Part model, mm, in its own coordinate system. Face numbers are marked on the shaded views. A direction names the side the tool comes from. Give positions to 0.01 mm unless a question says otherwise; leave off trailing zeros. Order: outer loops, then holes, each group sorted by start corner. A loop starts at its lowest first (then second) coordinate and runs counter-clockwise, first axis right, second up.
1. Probe line 1 (Y direction, x = -3.3, z = 7); line 2 (X direction, y = 2.5, z = -8.25); line 3 (X direction, y = 2, z = 7.5). List the from-to ranges inside material, lowest first.
2. Which spindle directions (+Z, -Z, +X, -X, +Y, -Y) get a long thin tool onto all of the face, cutting with end or side? Do the marked faces 1, 2 and 3. Say none if no direction does.
3. Slice it at A-A on z = 5. List the corners of the cut face in (x, y).
4. Mould opens along X. For the marked faces 4, 5, 6 and 7 say: +X half, -X half, draft (parallel to the pull), parting line (faces both ways), or undercut.
5. Drop flat-ended pins along their axis: pin 1 Ø0.7 at (y, z) = (3, 0) entering from +X; pin 2 Ø4 at (y, z) = (5.5, 2.5) entering from +X; pin 3 Ø1.6 at (y, z) = (2, -0.5) entering from -X. Give the stop position or say it passes through.
6. Slice it at B-B on z = -3.75. List the corners of the cut face in (x, y).
7. Slice it at C-C on y = 7.5. Give the number of separate pieces and of enclosed holes in the cut face, and give its area (3 significant figures).
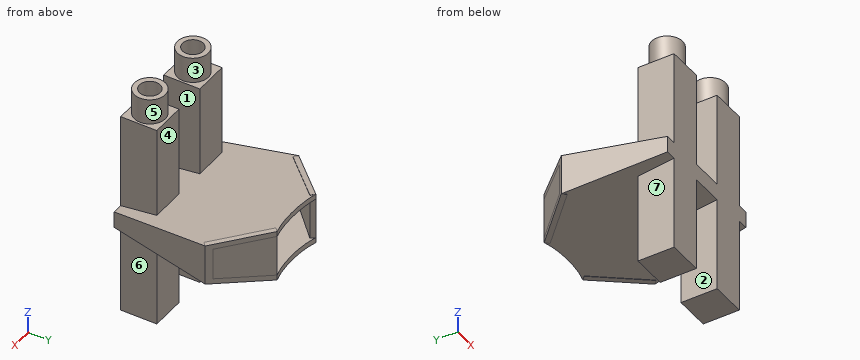
from build123d import *

# Parameters (mm, degrees)
SKETCH1_W                = 12
SKETCH1_H                = 1.6
BOSS_EXTRUDE1_DEPTH      = 15
BOSS_EXTRUDE1_TAPER      = -7
SHELL1_T                 = -0.5
SKETCH6_W                = 3.4
SKETCH6_H                = 20
BOSS_EXTRUDE2_DEPTH      = 3.5
BOSS_EXTRUDE2_2_DEPTH    = 3.5
CUT_EXTRUDE11_DEPTH      = 10
CUT_EXTRUDE11_DEPTH_BACK = 10
SKETCH11_RX              = 4.5
SKETCH11_RY              = 1.5
CUT_EXTRUDE12_DEPTH      = 10
BOSS_EXTRUDE3_DEPTH      = 0.5
SKETCH20_R               = 1.499118307
BOSS_EXTRUDE4_DEPTH      = 2.5
SKETCH22_R               = 1.001403974
CUT_EXTRUDE13_DEPTH      = 15
SKETCH25_W               = 2
SKETCH25_H               = 1.4
CUT_EXTRUDE14_DEPTH      = 1.5
SKETCH28_R               = 1.498355692
BOSS_EXTRUDE5_DEPTH      = 2.5
SKETCH29_R               = 1.002174376
CUT_EXTRUDE15_DEPTH      = 15
SKETCH30_W               = 3.2
SKETCH30_H               = 1.6
BOSS_EXTRUDE6_DEPTH      = 9
BOSS_EXTRUDE6_TAPER      = -6


with BuildPart() as part:
    # Sketch1 → Boss-Extrude1 (new body)
    with BuildSketch(Plane(origin=(0, 0, 0), x_dir=(1, 0, 0), z_dir=(0, 1, 0))):
        Rectangle(SKETCH1_W, SKETCH1_H)
    extrude(amount=BOSS_EXTRUDE1_DEPTH, taper=BOSS_EXTRUDE1_TAPER)

    # Shell1
    shell1_openings = [part.faces().sort_by_distance(p)[0] for p in [
        (0, 15, 0),
    ]]
    offset(amount=SHELL1_T, openings=shell1_openings, kind=Kind.INTERSECTION)

    # Sketch11 → Cut-Extrude11 (cut, two sides: drawn at the far end of the back side and taken through both)
    with BuildSketch(Plane.XY.offset(-CUT_EXTRUDE11_DEPTH_BACK)):
        with Locations((0, 15)):
            Ellipse(SKETCH11_RX, SKETCH11_RY)
    extrude(amount=CUT_EXTRUDE11_DEPTH + CUT_EXTRUDE11_DEPTH_BACK, mode=Mode.SUBTRACT)

    # Sketch18 → Cut-Extrude12 (cut, symmetric)
    with BuildSketch(Plane.XY):
        Polygon((-2.966549011, 13.872092056), (-7.173702506, 9.559039808), (-8.984967274, 15.813419698), (-2.966549011, 15.813419698), align=None)
    cut_extrude12 = extrude(amount=CUT_EXTRUDE12_DEPTH, both=True, mode=Mode.SUBTRACT)

    # Sketch19 → Boss-Extrude3 (add)
    with BuildSketch(Plane(origin=(-8.45404379, 8.246470904, 0), x_dir=(0, 0, 1), z_dir=(-0.7158402135047951, 0.6982641253346826, 0))):
        Polygon((1.973702506, 1.833605992), (2.503278732, 7.858766589), (-2.503278732, 7.858766589), (-1.973702506, 1.833605992), align=None)
    boss_extrude3 = extrude(amount=-BOSS_EXTRUDE3_DEPTH)

    # Mirror3: Boss-Extrude3 across plane
    add(boss_extrude3.mirror(Plane(origin=(0, 0, 0), x_dir=(0, 0, 1), z_dir=(1, 0, 0))))


with BuildPart() as body_2:
    # Sketch6 → Boss-Extrude2 (new body)
    with BuildSketch(Plane.XZ):
        with Locations((-3.3, 0)):
            Rectangle(SKETCH6_W, SKETCH6_H)
    extrude(amount=-BOSS_EXTRUDE2_DEPTH)


with BuildPart() as body_3:
    # Sketch6 → Boss-Extrude2 2 (new body)
    with BuildSketch(Plane.XZ):
        with Locations((3.3, 0)):
            Rectangle(SKETCH6_W, SKETCH6_H)
    extrude(amount=-BOSS_EXTRUDE2_2_DEPTH)

    # Sketch20 → Boss-Extrude4 (add)
    with BuildSketch(Plane.XY.offset(10)):
        with Locations((3.3, 1.75)):
            Circle(SKETCH20_R)
    extrude(amount=BOSS_EXTRUDE4_DEPTH)


with BuildPart() as cut_extrude13_tool:
    # Sketch22 → Cut-Extrude13 (new body)
    with BuildSketch(Plane.XY.offset(12.5)):
        with Locations((3.3, 1.75)):
            Circle(SKETCH22_R)
    extrude(amount=-CUT_EXTRUDE13_DEPTH)


with BuildPart() as part_1:
    add(part.part)

    # Cut-Extrude13: cut by cut_extrude13_tool
    add(cut_extrude13_tool.part, mode=Mode.SUBTRACT)


with BuildPart() as body_3_1:
    add(body_3.part)

    # Cut-Extrude13: cut by cut_extrude13_tool
    add(cut_extrude13_tool.part, mode=Mode.SUBTRACT)


with BuildPart() as cut_extrude14_tool:
    # Sketch25 → Cut-Extrude14 (new body)
    with BuildSketch(Plane(origin=(0, 3.5, 0), x_dir=(1, 0, 0), z_dir=(0, 1, 0))):
        with Locations((-3.371950412, 0.026080252)):
            Rectangle(SKETCH25_W, SKETCH25_H)
    cut_extrude14 = extrude(amount=-CUT_EXTRUDE14_DEPTH)


with BuildPart() as part_2:
    add(part_1.part)

    # Cut-Extrude14: cut by cut_extrude14_tool
    add(cut_extrude14_tool.part, mode=Mode.SUBTRACT)


with BuildPart() as body_2_1:
    add(body_2.part)

    # Cut-Extrude14: cut by cut_extrude14_tool
    add(cut_extrude14_tool.part, mode=Mode.SUBTRACT)

    # Sketch28 → Boss-Extrude5 (add)
    with BuildSketch(Plane.XY.offset(10)):
        with Locations((-3.3, 1.75)):
            Circle(SKETCH28_R)
    extrude(amount=BOSS_EXTRUDE5_DEPTH)


with BuildPart() as mirror6_tool:
    # Mirror6: Cut-Extrude14 across plane
    add(cut_extrude14.mirror(Plane(origin=(0, 0, 0), x_dir=(0, 0, 1), z_dir=(1, 0, 0))))


with BuildPart() as part_3:
    add(part_2.part)

    # Mirror6: cut by mirror6_tool
    add(mirror6_tool.part, mode=Mode.SUBTRACT)


with BuildPart() as body_3_2:
    add(body_3_1.part)

    # Mirror6: cut by mirror6_tool
    add(mirror6_tool.part, mode=Mode.SUBTRACT)


with BuildPart() as cut_extrude15_tool:
    # Sketch29 → Cut-Extrude15 (new body)
    with BuildSketch(Plane.XY.offset(12.5)):
        with Locations((-3.3, 1.75)):
            Circle(SKETCH29_R)
    extrude(amount=-CUT_EXTRUDE15_DEPTH)


with BuildPart() as part_4:
    add(part_3.part)

    # Cut-Extrude15: cut by cut_extrude15_tool
    add(cut_extrude15_tool.part, mode=Mode.SUBTRACT)



with BuildPart() as body_2_2:
    add(body_2_1.part)

    # Cut-Extrude15: cut by cut_extrude15_tool
    add(cut_extrude15_tool.part, mode=Mode.SUBTRACT)


with BuildPart() as part_5:
    add(part_4.part)

    add(body_2_2.part)  # Boss-Extrude6 merges body 2

    add(body_3_2.part)  # Boss-Extrude6 merges body 3
    # Sketch30 → Boss-Extrude6 (add)
    with BuildSketch(Plane.XZ):
        Rectangle(SKETCH30_W, SKETCH30_H)
    extrude(amount=-BOSS_EXTRUDE6_DEPTH, taper=BOSS_EXTRUDE6_TAPER)

    # Mirror7: Cut-Extrude12 across plane
    add(cut_extrude12.mirror(Plane(origin=(0, 0, 0), x_dir=(0, 0, 1), z_dir=(1, 0, 0))), mode=Mode.SUBTRACT)


solid = part_5.part
Data:
1. line 1: y = 0 to 0.75, 2.75 to 3.5
1. line 2: x = -5 to -1.6, 1.6 to 5
1. line 3: x = -5 to -4.27, -2.33 to -1.6, 1.6 to 2.33, 4.27 to 5
2. face 1: +Z, -Y
2. face 2: -Z, -Y
2. face 3: +Z
3. outline: (-5, 0) - (-1.6, 0) - (-1.6, 3.5) - (-5, 3.5) - close; (1.6, 0) - (5, 0) - (5, 3.5) - (1.6, 3.5) - close; hole circle Ø2 at (-3.3, 1.75); hole circle Ø2 at (3.3, 1.75)
4. face 4: draft
4. face 5: undercut
4. face 6: +X half
4. face 7: -X half
5. pin 1: stops at x = 6.41
5. pin 2: stops at x = 6.9
5. pin 3: stops at x = -6.34
6. outline: (-5, 0) - (-1.6, 0) - (-1.6, 3.5) - (-5, 3.5) - close; (1.6, 0) - (5, 0) - (5, 3.5) - (1.6, 3.5) - close
7. separate pieces: 1
7. enclosed holes: 2
7. area: 28.0 mm2
